Study the drawing (mm; zero at the part's minimum x, y, z) and answer. A direction names the side the tool comes from. Give positions to 0.01 mm unless a question says otherwise; leave off trailing zeros. Order: outer loops, then holes, each group sorted by start corner. A loop starts at its lowest first (then second) coordinate and runs counter-clockwise, first axis right, second up. Notation, with made-up numbers: (-6.75, 86.5) - (0.25, 86.5) arc R22 cw to (0.25, 120.5) - close; hole circle Ø10 at (-26, 0). An arc over 180 degrees is marked (long way). Put each result on its own line as item: value.
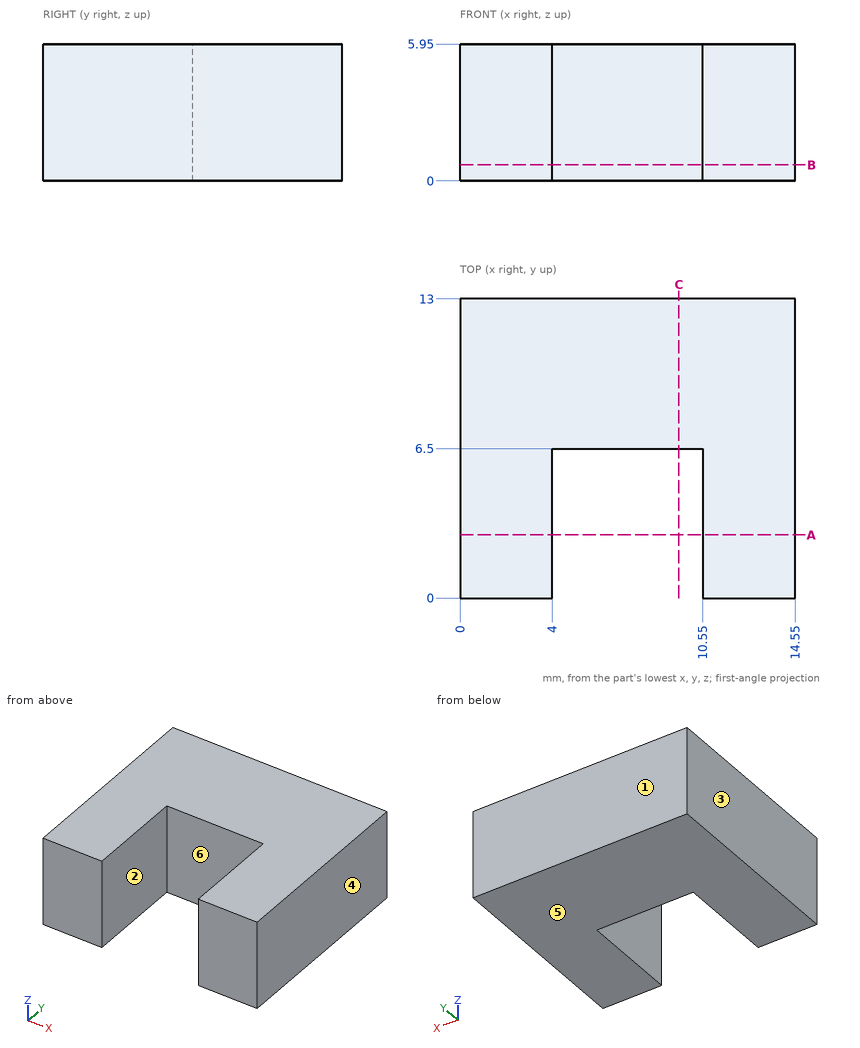
(1) A tool of negligible diameter and unlimited length cuts with its end or side. For the marked faces 1 and 2, from which of +Z, -Z, +X, -X, +Y, -Y can it reach the whole face along a straight path? Write none if from no direction.
Geometry check:
face 1: +Z, -Z, +X, -X, +Y
face 2: +Z, -Z, -Y
(2) Determine the mould class of the marked faces 3, 4, 5 and 6 for opening direction X: pulls with the +X half, pulls with the -X half, needs draft (parallel to the pull), parting line crosses it, or undercut.
Geometry check:
face 3: pulls with the -X half
face 4: pulls with the +X half
face 5: needs draft
face 6: undercut
(3) Section A-A, the plane y = 2.75 is taken. Write down the section's boundary in (x, z).
Geometry check:
outline: (0, 0) - (4, 0) - (4, 5.95) - (0, 5.95) - close; (10.55, 0) - (14.55, 0) - (14.55, 5.95) - (10.55, 5.95) - close
(4) Section C-C, the plane x = 9.5 is taken. Write down the section's boundary in (y, z), then the cut area to 3 significant figures.
Geometry check:
outline: (6.5, 0) - (13, 0) - (13, 5.95) - (6.5, 5.95) - close
area: 38.7 mm²
(5) Section B-B, the plane z = 0.7 is taken. Write down the section's boundary in (x, y).
Geometry check:
outline: (0, 0) - (4, 0) - (4, 6.5) - (10.55, 6.5) - (10.55, 0) - (14.55, 0) - (14.55, 13) - (0, 13) - close
(6) Straight lines are drawn through the part: line 1 (X direction, y = 1, z = 3.85); line 2 (Y direction, x = 6.25, z = 3.45). For each, find the intervals that lie inside material, in ascending order.
Geometry check:
line 1: x = 0 to 4, 10.55 to 14.55
line 2: y = 6.5 to 13
